Here's how the part is built. I have some questions about the finished solid (model axes, mm). Give positions to 0.01 mm unless a question says otherwise; leave off trailing zeros. Write each loop counter-clockwise with the first axis right and the second up, starting at its lowest first coordinate (ties: lowest second). Pieces come first, ordered by that corner, then holes. Notation, with made-up numbers: (-30.75, 82.25) -> (0.25, 82.25) arc R10 cw to (0.25, 97.25) -> close; hole circle Ø11 at (-36, 21.5). An arc over 180 degrees is marked (long way). Use CSV: the item, a comma, the result in double quotes. Start each with the question number.
(1) Suppose I cut it at A-A on y = 20. List the corners of the cut face in (x, z) for me, plus the area to 3 significant figures.
(2) I need wall thicknesses on L1, parallel to Y at x = -20, z = 0.7; L2, parallel to Y at x = -31, z = 1.6; L3, parallel to X at y = 32, z = 1.1. Which ranges of each line are inside material? Lowest first, please. Write a range as [from, to].
(3) Suppose I cut it at C-C on y = -31. Give the number of separate pieces and of enclosed holes in the cut face, plus the area to 3 significant figures.
(4) Suppose I cut it at B-B on x = -31. List the corners of the cut face in (y, z) for me.
(5) For pin 1 Ø4 at (x, y) = (-31, 31) entering from +Z; pin 2 Ø11 at (x, y) = (31, 31) entering from +Z, each with a flat end and sliding along its axis, tell me the tip position at first contact or that it passes through.
from build123d import *

# Parameters (mm, degrees)
F0_W        = 76
F0_H        = 76
F0_R        = 6
F0_R_2      = 1.5
F0_W_2      = 7
F0_H_2      = 18
F1_DEPTH    = 3
F0_R_3      = 3.5
F2_DEPTH    = 1
F3_T1_DEPTH = 3
F3_T3_DEPTH = 28
F4_R        = 0.5


# Not quite as in the source:
# - a fillet or chamfer that OpenCascade refuses, or shapes differently, is made with other operations: its cross-section is extruded or revolved along the edge and cut away or added
# - a feature names something its author has since deleted; it is built from what else it names


with BuildPart() as f1:
    # F0 (on Top) → F1 (new body)
    with BuildSketch(Plane.XY):
        Rectangle(F0_W, F0_H)
        with Locations((-31, -31)):
            Circle(F0_R, mode=Mode.SUBTRACT)
        with Locations((-20, -20)):
            Circle(F0_R_2, mode=Mode.SUBTRACT)
        with Locations((0, -31)):
            Circle(F0_R, mode=Mode.SUBTRACT)
        with Locations((31, -31)):
            Circle(F0_R, mode=Mode.SUBTRACT)
        with Locations((20, -20)):
            Circle(F0_R_2, mode=Mode.SUBTRACT)
        with Locations((-20, 20)):
            Circle(F0_R_2, mode=Mode.SUBTRACT)
        with Locations((-31, 31)):
            Circle(F0_R, mode=Mode.SUBTRACT)
        with Locations((31, 0)):
            Rectangle(F0_W_2, F0_H_2, mode=Mode.SUBTRACT)
        with Locations((0, 31)):
            Circle(F0_R, mode=Mode.SUBTRACT)
        with Locations((20, 20)):
            Circle(F0_R_2, mode=Mode.SUBTRACT)
        with Locations((31, 31)):
            Circle(F0_R, mode=Mode.SUBTRACT)
    extrude(amount=F1_DEPTH)

    # F0 (on Top) → F2 (join)
    with BuildSketch(Plane.XY):
        with Locations((-31, 31)):
            Circle(F0_R)
        with Locations((-31, 31)):
            Circle(F0_R_3, mode=Mode.SUBTRACT)
        with Locations((31, 31)):
            Circle(F0_R)
        with Locations((31, 31)):
            Circle(F0_R_3, mode=Mode.SUBTRACT)
        with Locations((31, -31)):
            Circle(F0_R)
        with Locations((31, -31)):
            Circle(F0_R_3, mode=Mode.SUBTRACT)
        with Locations((-31, -31)):
            Circle(F0_R)
        with Locations((-31, -31)):
            Circle(F0_R_3, mode=Mode.SUBTRACT)
        with Locations((0, 31)):
            Circle(F0_R)
        with Locations((0, 31)):
            Circle(F0_R_3, mode=Mode.SUBTRACT)
        with Locations((0, -31)):
            Circle(F0_R)
        with Locations((0, -31)):
            Circle(F0_R_3, mode=Mode.SUBTRACT)
    extrude(amount=F2_DEPTH)

    # F3: fillet of radius 5 on 8 edges, made by hand

    # F3_s2 → F3_t1 (join)
    with BuildSketch(Plane.XY):
        with BuildLine():
            ThreePointArc((29.5, 9), (33.0355339059, 7.5355339059), (34.5, 4))
            Line((34.5, 4), (34.5, 9))
            Line((34.5, 9), (29.5, 9))
        make_face()
        with BuildLine():
            ThreePointArc((29.5, -9), (33.0355339059, -7.5355339059), (34.5, -4))
            Line((34.5, -4), (34.5, -9))
            Line((34.5, -9), (29.5, -9))
        make_face()
        with BuildLine():
            ThreePointArc((32.5, -9), (28.9644660941, -7.5355339059), (27.5, -4))
            Line((27.5, -4), (27.5, -9))
            Line((27.5, -9), (32.5, -9))
        make_face()
        with BuildLine():
            ThreePointArc((27.5, 4), (28.9644660941, 7.5355339059), (32.5, 9))
            Line((32.5, 9), (27.5, 9))
            Line((27.5, 9), (27.5, 4))
        make_face()
    extrude(amount=F3_T1_DEPTH)

    # F3_s4 → F3_t3 (cut)
    with BuildSketch(Plane.XY.offset(-12.5)):
        with BuildLine():
            ThreePointArc((-33, -38), (-36.5355339059, -36.5355339059), (-38, -33))
            Line((-38, -33), (-38, -38))
            Line((-38, -38), (-33, -38))
        make_face()
        with BuildLine():
            ThreePointArc((33, -38), (36.5355339059, -36.5355339059), (38, -33))
            Line((38, -33), (38, -38))
            Line((38, -38), (33, -38))
        make_face()
        with BuildLine():
            ThreePointArc((38, 33), (36.5355339059, 36.5355339059), (33, 38))
            Line((33, 38), (38, 38))
            Line((38, 38), (38, 33))
        make_face()
        with BuildLine():
            ThreePointArc((-38, 33), (-36.5355339059, 36.5355339059), (-33, 38))
            Line((-33, 38), (-38, 38))
            Line((-38, 38), (-38, 33))
        make_face()
    extrude(amount=F3_T3_DEPTH, mode=Mode.SUBTRACT)

    # F4
    f4_edges = [f1.edges().sort_by_distance(p)[0] for p in [
        (0, -38, 3),
    ]]
    fillet(f4_edges, radius=F4_R)


solid = f1.part
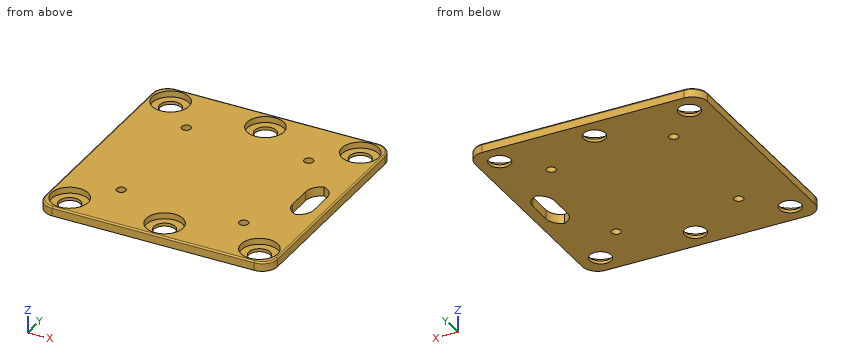
Geometry says:
1,outline,"(-38, 0) -> (-21.5, 0) -> (-21.5, 3) -> (-37.5, 3) arc R0.5 ccw to (-38, 2.5) -> close; (-18.5, 0) -> (18.5, 0) -> (18.5, 3) -> (-18.5, 3) -> close; (21.5, 0) -> (38, 0) -> (38, 2.5) arc R0.5 ccw to (37.5, 3) -> (21.5, 3) -> close"
1,area,"210 mm²"
2,L1,"[-38, -21.5], [-18.5, 18.5], [21.5, 38]"
2,L2,"[-38, -37], [-25, 25], [37, 38]"
2,L3,"[-38, -36.92], [-25.08, -5.92], [5.92, 25.08], [36.92, 38]"
3,separate pieces,"4"
3,enclosed holes,"0"
3,area,"135 mm²"
4,outline,"(-38, 0) -> (-34.5, 0) -> (-34.5, 1) -> (-37, 1) -> (-37, 3) -> (-37.5, 3) arc R0.5 ccw to (-38, 2.5) -> close; (-27.5, 0) -> (27.5, 0) -> (27.5, 1) -> (25, 1) -> (25, 3) -> (-25, 3) -> (-25, 1) -> (-27.5, 1) -> close; (34.5, 0) -> (38, 0) -> (38, 2.5) arc R0.5 ccw to (37.5, 3) -> (37, 3) -> (37, 1) -> (34.5, 1) -> close"
5,pin 1,"through"
5,pin 2,"z = 1"
